Work out the finished part from the listing and answer in its coordinate system (mm). Face numbers are marked on the shaded views. A direction names the side the tool comes from. Give positions to 0.01 mm unless a question says otherwise; leave off trailing zeros. Write each loop counter-clockwise with the first axis right and the second up, starting at its lowest first coordinate (ties: lowest second). Pieces come first, ordered by that corner, then holes. Notation, with made-up numbers: (33, -36.5) - (82, -36.5) arc R27 ccw to (82, 2.5) - close; hole circle Ø1 at (87.5, 1.25). An arc over 180 degrees is marked (long way). Write item = value, one per line.
Autodesk Inventor part; units mm, degrees
ref_plane "Work Plane2" through (0, 0, 3.5) normal (0, 0, 1) x (1, 0, 0)
ref_plane "Work Plane8" through (0, 0, 0) normal (0.9396926, 0.3420201, 0) x (0, 0, 1)
ref_plane "Work Plane9" through (0, 0, 0) normal (1, 0, 0) x (0, 1, 0)
sketch "Sketch1" plane through (0, 0, 0) normal (0, 0, 1) x (1, 0, 0)
  circle A0 centre (0, 0) radius 16.4816
  dimension "d0" = 32.9631
extrude "Extrusion1" add sketch "Sketch1" along normal blind 7
ref_plane "Work Plane2" through (0, 0, 3.5) normal (0, 0, 1) x (1, 0, 0)
sketch "Sketch2" plane through (0, 0, 0) normal (0, 0, -1) x (-1, 0, 0)
  circle A0 centre (0, 0) radius 16.4816
  circle A1 centre (0, 0) radius 13.5
  dimension "d3" = 27
surface extrude "Pitch Diameter" sketch "Sketch2" against normal through all shown no curves A1
ref_plane "Work Plane8" through (0, 0, 0) normal (0.9396926, 0.3420201, 0) x (0, 0, 1)
ref_plane "Work Plane9" through (0, 0, 0) normal (1, 0, 0) x (0, 1, 0)
spur gear teeth "Spur Gear" teeth 9 pitch diameter 27 tip diameter 32.9632 root diameter 19.5 face width 7 start plane through (0, 0, 0) normal (0, 0, -1) x (-1, 0, 0)
sketch "Sketch3" plane through (0, 0, 7) normal (0, 0, 1) x (1, 0, 0)
  point P0 (0, 0)
sketch "Sketch4" plane through (0, 0, 7) normal (0, 0, 1) x (1, 0, 0)
  circle A0 centre (0, 0) radius 4.15
  dimension "d49" = 8.3
extrude "Extrusion2" cut sketch "Sketch4" against normal blind 10
equation "\"d0\" = da_da"
equation "\"d1\" = da_b"
equation "\"d3\" = da_d"
properties part number "Spur Gear1" material "Steel"
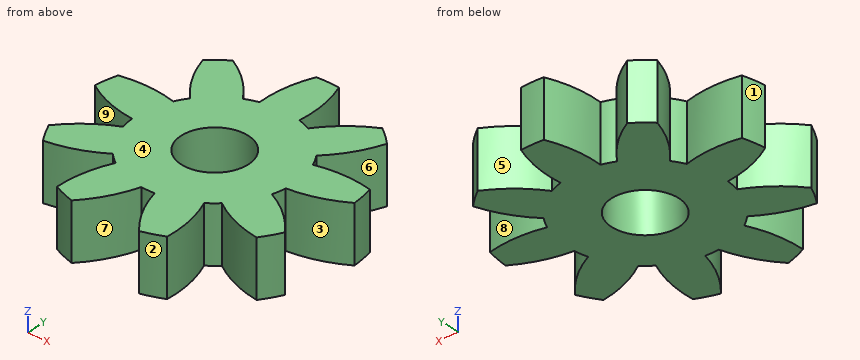
1. Find section B-B, the plane y = -2. Give the vertices of the cut face in (x, z), then the cut area to 3 significant figures.
Solution:
outline = (-9.54, 0) - (-3.64, 0) - (-3.64, 7) - (-9.54, 7) - close; (3.64, 0) - (9.54, 0) - (9.54, 7) - (3.64, 7) - close
area = 82.7 mm^2
2. Straight lines are drawn through the part: line 1 (X direction, y = 11.5, z = 2.5); line 2 (X direction, y = 11, z = 2); line 3 (Y direction, x = -9, z = 3). For each, find the intervals that lie inside material, in ascending order.
Solution:
line_1 = -11.6 to -6.53, -2.55 to 2.55, 6.53 to 11.6
line_2 = -11.43 to -5.99, -2.57 to 2.57, 5.99 to 11.43
line_3 = -8.11 to 4.16, 6.73 to 13.25
3. Find section C-C, the plane x = -11. Give the vertices of the cut face in (y, z), then the cut area to 3 significant figures.
Solution:
outline = (-8.9, 0) - (-3.39, 0) - (-3.39, 7) - (-8.9, 7) - close; (-0.67, 0) - (4.52, 0) - (4.52, 7) - (-0.67, 7) - close; (9.96, 0) - (12.27, 0) - (12.27, 7) - (9.96, 7) - close
area = 91.1 mm^2
4. Given pin 1 (2 mm diameter, centred on x = -12.5, z = 3.5, fed in from +Y); pin 2 (4 mm diameter, centred on y = 10.5, z = 6.5, fed in from -X), each flat-ended and moving along its own axis, determine where each tip first touches the part or whether it passes through.
Solution:
pin_1 = 11.81
pin_2 = -11.65
5. Find section A-A, the plane x = 0. Give the vertices of the cut face in (y, z), then the cut area to 3 significant figures.
Solution:
outline = (-9.75, 0) - (-4.15, 0) - (-4.15, 7) - (-9.75, 7) - close; (4.15, 0) - (16.48, 0) - (16.48, 7) - (4.15, 7) - close
area = 126 mm^2
6. For a pull along Y with two mould halves and no side action, classify the marked faces 1, 2, 3 and 4 as pulls with the +Y half, pulls with the -Y half, needs draft (parallel to the pull), parting line crosses it, or undercut.
Solution:
face_1 = pulls with the +Y half
face_2 = pulls with the -Y half
face_3 = undercut
face_4 = needs draft
7. Find section D-D, the plane y = -6.5. Give the vertices of the cut face in (x, z), then the cut area to 3 significant figures.
Solution:
outline = (-14.56, 0) - (14.56, 0) - (14.56, 7) - (-14.56, 7) - close
area = 204 mm^2
8. A tool of negligible diameter and unlimited length cuts with its end or side. For the marked faces 5, 6, 7, 8 and 9, from which of +Z, -Z, +X, -X, +Y, -Y can it reach the whole face along a straight path? Write none if from no direction.
Solution:
face_5 = +Z, -Z, +Y
face_6 = +Z, -Z, +X
face_7 = +Z, -Z, -Y
face_8 = +Z, -Z
face_9 = +Z, -Z, -X
